Geometry: final body of the model. Coordinates: model frame, mm. A direction names the side the tool comes from. Give positions to 0.01 mm unless a question says otherwise; leave off trailing zeros. Write each loop counter-clockwise with the first axis right and the second up, starting at its lowest first coordinate (ties: lowest second). Pieces come first, ordered by that corner, then holes.
Q1. Cut plane A-A on x = 69. Return the cut outline in (y, z).
Q2. Cut plane B-B on y = 24. Return the cut outline in (x, z).
Q3. Cut plane D-D on y = 57.5. Return the cut outline in (x, z) (3 decimals), plus the area to 3 significant figures.
Q4. Draft query along Z for faces 5 (the face through (34, 55.75, 34)), 6 (the face through (15.9, 10.5, 31.6)), 7 (the face through (13.314, 10.246, 31.425)). Return one class per face: pulls with the +Z half, pulls with the -Z half, needs draft (parallel to the pull), parting line crosses it, or undercut.
Q5. Pin query (flat end, axial travel): pin 1 (6 mm diameter, centred on y = 45.5, z = 26, fed in from -X); pin 2 (2.5 mm diameter, centred on x = 6, z = 32, fed in from +Y); pin 3 (12 mm diameter, centred on x = 57.5, y = 57.5, fed in from -Z). Return the tip coordinate at first contact, or that it passes through.
Q6. Reachability of faces 1 (the face through (28.77, 46.48, 54.66)), 2 (the face through (26, 40, 32)), 3 (the face through (61, 53, 30.09)), 4 (the face through (10, 51.25, 37)) from +Z, -Z, +X, -X, +Y, -Y: full face, straight path, thin tool, end or side. Return the list, or none.
Q7. Line query: L1, parallel to Y at x = 36.5, z = 10; L2, parallel to Y at x = 14, z = 29; L3, parallel to Y at x = 13, z = 17. Output: solid intervals per line, ascending.
Q8. Cut plane C-C on x = 6.5. Return the cut outline in (y, z), plus the area to 3 significant figures.
```python
from build123d import *

# Parameters (mm, degrees)
SKETCH1_W               = 80
SKETCH1_H               = 65
BOSS_EXTRUDE1_DEPTH     = 65
SKETCH3_W               = 22
SKETCH3_H               = 15.09
CUT_EXTRUDE1_DEPTH      = 65.72
CUT_EXTRUDE2_DEPTH      = 20
CUT_EXTRUDE2_DEPTH_BACK = 55.72
SKETCH4_R               = 2.245
SKETCH4_R_2             = 2.24505
SKETCH5_W               = 65
SKETCH5_H               = 10
SKETCH5_H_2             = 2
CUT_EXTRUDE3_DEPTH      = 40
CUT_EXTRUDE4_DEPTH      = 65
SKETCH10_R              = 1
CUT_EXTRUDE6_DEPTH      = 42
SKETCH12_R              = 2.9
SKETCH12_R_2            = 6
CUT_EXTRUDE7_DEPTH      = 20
SKETCH14_W              = 23
SKETCH14_H              = 12.5
CUT_EXTRUDE9_DEPTH      = 13.75
SKETCH16_W              = 5
SKETCH16_H              = 12.5
SKETCH16_R              = 1.25
CUT_EXTRUDE10_DEPTH     = 9.25
SKETCH16_4_R            = 1.25
CUT_EXTRUDE11_DEPTH     = 12.5
CUT_EXTRUDE12_DEPTH     = 21.5
CUT_EXTRUDE13_DEPTH     = 8
SKETCH20_R              = 2
BOSS_EXTRUDE2_DEPTH     = 0.5
SKETCH21_R              = 2
BOSS_EXTRUDE3_DEPTH     = 0.5
SKETCH22_R              = 1
CUT_EXTRUDE14_DEPTH     = 30.5
SKETCH23_W              = 37
SKETCH23_H              = 30.09
CUT_EXTRUDE15_DEPTH     = 24


with BuildPart() as part:
    # Sketch1 → Boss-Extrude1 (new body)
    with BuildSketch(Plane.XY):
        with Locations((40, 32.5)):
            Rectangle(SKETCH1_W, SKETCH1_H)
    extrude(amount=BOSS_EXTRUDE1_DEPTH)

    # Sketch3 → Cut-Extrude1 (cut)
    with BuildSketch(Plane.XZ):
        with Locations((69, 57.455)):
            Rectangle(SKETCH3_W, SKETCH3_H)
        with Locations((69, 7.545)):
            Rectangle(SKETCH3_W, SKETCH3_H)
    extrude(amount=-CUT_EXTRUDE1_DEPTH, mode=Mode.SUBTRACT)

    # Sketch4 → Cut-Extrude2 (cut, two sides: drawn at the far end of the back side and taken through both)
    with BuildSketch(Plane.XY.offset(49.91).offset(-CUT_EXTRUDE2_DEPTH_BACK)):
        with Locations(Location((54, 57.5, 0), (0, 0, 180))):
            Circle(SKETCH4_R)
        with Locations(Location((69, 7.5, 0), (0, 0, 180))):
            Circle(SKETCH4_R_2)
    extrude(amount=CUT_EXTRUDE2_DEPTH + CUT_EXTRUDE2_DEPTH_BACK, mode=Mode.SUBTRACT)

    # Sketch5 → Cut-Extrude3 (cut)
    with BuildSketch(Plane.ZY):
        with Locations((32.5, 35)):
            Rectangle(SKETCH5_W, SKETCH5_H)
        with Locations((32.5, 15)):
            Rectangle(SKETCH5_W, SKETCH5_H)
        with Locations((32.5, 44)):
            Rectangle(SKETCH5_W, SKETCH5_H_2)
    extrude(amount=-CUT_EXTRUDE3_DEPTH, mode=Mode.SUBTRACT)

    # Sketch6 → Cut-Extrude4 (cut)
    with BuildSketch(Plane.XZ):
        with BuildLine():
            Line((0, 0), (43, 0))
            Line((43, 0), (7.776682895, 19.353757571))
            ThreePointArc((7.776682895, 19.353757571), (2.089737482, 24.862911437), (0, 32.5))
            Line((0, 32.5), (0, 0))
        make_face()
        with BuildLine():
            Line((0, 65), (0, 32.5))
            ThreePointArc((0, 32.5), (2.089737482, 40.137088563), (7.776682895, 45.646242429))
            Line((7.776682895, 45.646242429), (43, 65))
            Line((43, 65), (0, 65))
        make_face()
    extrude(amount=-CUT_EXTRUDE4_DEPTH, mode=Mode.SUBTRACT)

    # Sketch10 → Cut-Extrude6 (cut)
    with BuildSketch(Plane.XZ):
        with Locations(Location((15, 32.5, 0), (0, 0, 270))):
            Circle(SKETCH10_R)
    extrude(amount=-CUT_EXTRUDE6_DEPTH, mode=Mode.SUBTRACT)

    # Sketch12 → Cut-Extrude7 (cut)
    with BuildSketch(Plane(origin=(0, 65, 0), x_dir=(1, 0, 0), z_dir=(0, 1, 0))):
        with Locations((21.452618395, -32.5)):
            Circle(SKETCH12_R)
        with Locations((15, -32.5)):
            Circle(SKETCH12_R_2)
        with BuildLine():
            Line((21.452618395, -29.6), (20.252618395, -29.6))
            ThreePointArc((20.252618395, -29.6), (20.309467908, -29.705442695), (20.364201004, -29.811999333))
            ThreePointArc((20.364201004, -29.811999333), (20.898182616, -29.653493199), (21.452618395, -29.6))
        make_face()
        with BuildLine():
            ThreePointArc((20.364201004, -35.188000667), (20.309467908, -35.294557305), (20.252618395, -35.4))
            Line((20.252618395, -35.4), (21.452618395, -35.4))
            ThreePointArc((21.452618395, -35.4), (20.898182616, -35.346506801), (20.364201004, -35.188000667))
        make_face()
    extrude(amount=-CUT_EXTRUDE7_DEPTH, mode=Mode.SUBTRACT)

    # Sketch14 → Cut-Extrude9 (cut)
    with BuildSketch(Plane(origin=(0, 65, 0), x_dir=(1, 0, 0), z_dir=(0, 1, 0))):
        with Locations((20.5, -32.5)):
            Rectangle(SKETCH14_W, SKETCH14_H)
    extrude(amount=-CUT_EXTRUDE9_DEPTH, mode=Mode.SUBTRACT)

    # Sketch16 → Cut-Extrude10 (cut)
    # profile 1 of 4: a face of its own
    with BuildSketch(Plane(origin=(0, 65, 0), x_dir=(1, 0, 0), z_dir=(0, 1, 0))):
        with Locations((6.5, -32.5)):
            Rectangle(SKETCH16_W, SKETCH16_H)
        with Locations((6.5, -32.5)):
            Circle(SKETCH16_R, mode=Mode.SUBTRACT)
    # profile 2 of 4: a face of its own
    with BuildSketch(Plane(origin=(0, 65, 0), x_dir=(1, 0, 0), z_dir=(0, 1, 0))):
        with Locations((6.5, -32.5)):
            Circle(SKETCH16_R)
    # profile 3 of 4: a face of its own
    with BuildSketch(Plane(origin=(0, 65, 0), x_dir=(1, 0, 0), z_dir=(0, 1, 0))):
        with Locations((34.5, -32.5)):
            Rectangle(SKETCH16_W, SKETCH16_H)
        with Locations((34.5, -32.5)):
            Circle(SKETCH16_R, mode=Mode.SUBTRACT)
    # profile 4 of 4: a face of its own
    with BuildSketch(Plane(origin=(0, 65, 0), x_dir=(1, 0, 0), z_dir=(0, 1, 0))):
        with Locations((34.5, -32.5)):
            Circle(SKETCH16_R)
    extrude(amount=-CUT_EXTRUDE10_DEPTH, mode=Mode.SUBTRACT)

    # Sketch16<4> → Cut-Extrude11 (cut)
    with BuildSketch(Plane(origin=(0, 65, 0), x_dir=(1, 0, 0), z_dir=(0, 1, 0))):
        with Locations(Location((6.5, -32.5, 0), (0, 0, 270))):
            Circle(SKETCH16_4_R)
        with Locations(Location((34.5, -32.5, 0), (0, 0, 270))):
            Circle(SKETCH16_4_R)
    extrude(amount=-CUT_EXTRUDE11_DEPTH, mode=Mode.SUBTRACT)

    # Sketch18 → Cut-Extrude12 (cut)
    with BuildSketch(Plane(origin=(0, 65, 0), x_dir=(1, 0, 0), z_dir=(0, 1, 0))):
        with BuildLine():
            ThreePointArc((18.531385071, -32.863069526), (15, -36.05), (11.468614929, -32.863069526))
            Line((11.468614929, -32.863069526), (11.770443602, -38.75))
            Line((11.770443602, -38.75), (18.229556398, -38.75))
            Line((18.229556398, -38.75), (18.531385071, -32.863069526))
        make_face()
        with BuildLine():
            Line((15.593717104, -29), (14.406282896, -29))
            ThreePointArc((14.406282896, -29), (12.287971634, -30.209279122), (11.45, -32.5))
            Line((11.45, -32.5), (11.468614929, -32.863069526))
            ThreePointArc((11.468614929, -32.863069526), (15, -36.05), (18.531385071, -32.863069526))
            Line((18.531385071, -32.863069526), (18.55, -32.5))
            ThreePointArc((18.55, -32.5), (17.712028366, -30.209279122), (15.593717104, -29))
        make_face()
        with BuildLine():
            ThreePointArc((15.593717104, -29), (15, -28.95), (14.406282896, -29))
            Line((14.406282896, -29), (15.593717104, -29))
        make_face()
        Polygon((18.229556398, -38.75), (11.770443602, -38.75), (12.25004092, -48.104167856), (17.599264584, -51.043345268), align=None)
    extrude(amount=-CUT_EXTRUDE12_DEPTH, mode=Mode.SUBTRACT)

    # Sketch19 → Cut-Extrude13 (cut)
    with BuildSketch(Plane.XZ.offset(-40)):
        with BuildLine():
            Line((15, 44), (40, 63.351623939))
            Line((40, 63.351623939), (7.776682895, 45.646242429))
            ThreePointArc((7.776682895, 45.646242429), (0, 32.5), (7.776682895, 19.353757571))
            Line((7.776682895, 19.353757571), (40, 1.648376061))
            Line((40, 1.648376061), (15, 21))
            ThreePointArc((15, 21), (3.5, 32.5), (15, 44))
        make_face()
    extrude(amount=-CUT_EXTRUDE13_DEPTH, mode=Mode.SUBTRACT)

    # Sketch20 → Boss-Extrude2 (add)
    with BuildSketch(Plane(origin=(0, 30, 0), x_dir=(1, 0, 0), z_dir=(0, 1, 0))):
        with Locations(Location((15, -32.5, 0), (0, 0, 90))):
            Circle(SKETCH20_R)
    extrude(amount=BOSS_EXTRUDE2_DEPTH)

    # Sketch21 → Boss-Extrude3 (add)
    with BuildSketch(Plane(origin=(0, 10, 0), x_dir=(1, 0, 0), z_dir=(0, 1, 0))):
        with Locations(Location((15, -32.5, 0), (0, 0, 90))):
            Circle(SKETCH21_R)
    extrude(amount=BOSS_EXTRUDE3_DEPTH)

    # Sketch22 → Cut-Extrude14 (cut)
    with BuildSketch(Plane.XZ):
        with Locations(Location((15, 32.5, 0), (0, 0, 270))):
            Circle(SKETCH22_R)
    extrude(amount=-CUT_EXTRUDE14_DEPTH, mode=Mode.SUBTRACT)

    # Sketch23 → Cut-Extrude15 (cut)
    with BuildSketch(Plane(origin=(0, 65, 0), x_dir=(1, 0, 0), z_dir=(0, 1, 0))):
        with Locations((61.5, -15.045)):
            Rectangle(SKETCH23_W, SKETCH23_H)
    extrude(amount=-CUT_EXTRUDE15_DEPTH, mode=Mode.SUBTRACT)


solid = part.part
```
Data:
1. outline: (0, 15.09) - (5.25, 15.09) - (5.25, 49.91) - (0, 49.91) - close; (9.75, 15.09) - (41, 15.09) - (41, 30.09) - (65, 30.09) - (65, 49.91) - (9.75, 49.91) - close
2. outline: (7.78, 19.35) - (43, 0) - (58, 0) - (58, 15.09) - (80, 15.09) - (80, 49.91) - (58, 49.91) - (58, 65) - (43, 65) - (7.78, 45.65) arc R15 ccw to start; hole circle Ø2 at (15, 32.5)
3. outline: (4, 26.25) - (4, 38.75) - (11.77, 38.75) - (12.25, 48.104) - (7.777, 45.646) arc R15 ccw to (7.777, 19.354) - (43, 0) - (43, 30.09) - (51.755, 30.09) - (51.755, 65) - (43, 65) - (17.599, 51.043) - (18.23, 38.75) - (37, 38.75) - (37, 26.25) - close; (56.245, 30.09) - (80, 30.09) - (80, 49.91) - (58, 49.91) - (58, 65) - (56.245, 65) - close
3. area: 2,080 mm2
4. face 5: undercut
4. face 6: needs draft
4. face 7: parting line crosses it
5. pin 1: stops at x = 0.8
5. pin 2: stops at y = 55.75
5. pin 3: stops at z = 30.09
6. face 1: +Z, -X
6. face 2: +Z, -Z, -X
6. face 3: -Z, +X, +Y
6. face 4: +Y
7. L1: y = 0 to 10, 20 to 30, 40 to 43, 45 to 65
7. L2: y = 0 to 10, 20 to 30, 40 to 43
7. L3: y = 0 to 10, 20 to 30, 48 to 65
8. outline: (0, 20.14) - (10, 20.14) - (10, 44.86) - (0, 44.86) - close; (20, 20.14) - (30, 20.14) - (30, 44.86) - (20, 44.86) - close; (40, 24.75) - (43, 24.75) - (43, 40.25) - (40, 40.25) - close; (45, 24.75) - (48, 24.75) - (48, 20.14) - (65, 20.14) - (65, 26.25) - (55.75, 26.25) - (55.75, 31.25) - (52.5, 31.25) - (52.5, 33.75) - (55.75, 33.75) - (55.75, 38.75) - (65, 38.75) - (65, 44.86) - (48, 44.86) - (48, 40.25) - (45, 40.25) - close
8. area: 884 mm2
